Autodesk Fusion 360 part; units mm, degrees
sketch "Sketch2" plane through (0, 0, 0) normal (1, 0, 0) x (0, 1, 0)
  circle A0 centre (73.75, 0) radius 21.29
  line L0 (0, 0) -> (147.5, 0) construction
  circle A1 centre (73.75, 0) radius 18.75
  line L1 (78.83, -20.32) -> (78.83, -17.78)
  circle A2 centre (0, 0) radius 35.49
  line L2 (35.49, 0) -> (52.46, 0)
  circle A3 centre (46.6735, 34.4155) radius 22.5
  circle A4 centre (46.6735, -34.4155) radius 22.5
  circle A5 centre (0, 0) radius 32.95
  dimension "d11" = 37.5
  dimension "d14" = 2.54
  dimension "d24" = 65.9
  dimension "d25" = 2.54
  dimension "d26" = 73.75
  dimension "d27" = 45
extrude "Extrude2" add sketch "Sketch2" along normal blind 15.24 contours A0 | A0 A2 L2 A3 | A0 A2 L2 A4 | A2
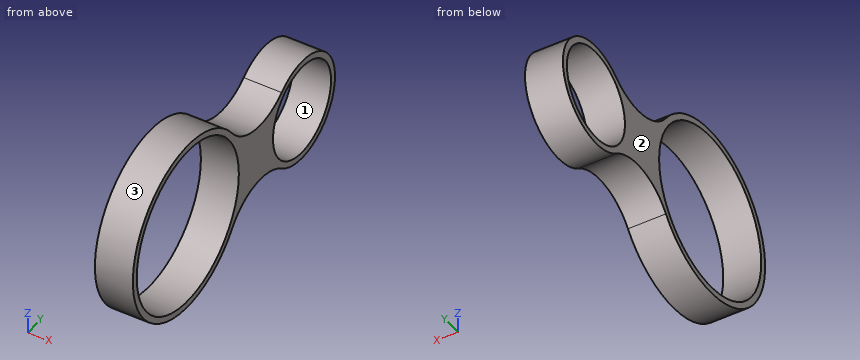
Can you work these out from the model? Positions are in its coordinate system, mm. Face numbers are marked on the shaded views. Give positions to 0.01 mm unless a question says otherwise; leave off trailing zeros. Loops run counter-clockwise (first coordinate to the right, second up) from the corner with the lowest first, then second, coordinate; pieces in that order, holes last. Notation, with made-up numbers: M -25.5,-21.75 L 26.5,-21.75 A24 ccw 26.5,9.25 Z; hole C -36.5,68 d9. An arc over 180 degrees is marked long. Use one line per item in the form item = value. Start each with the question number.
(1) I want a section at D-D, the plane x = 12.25. Write out the boundary of the cut face in (y, z), and give its area (3 significant figures).
(2) Thinking about a two-plate mould opening in Z: for the marked faces 1, 2 and 3, which applies, released by +Z, released by -Z, zero draft, split by the parting line, or undercut?
(3) I want a section at B-B, the plane y = 0. Write out the boundary of the cut face in (x, z), and give its area (3 significant figures).
(4) I'm going to push flat-ended pins straight in: P1, Ø6, axis at x = 10.5, z = 26, coming from the -Y side; P2, Ø3, axis at x = 4.5, y = 33, coming from the -Z side; P3, Ø6, axis at x = 9, z = -14, coming from the -Y side. Where does each tip first touch, or does it pass through?
(5) I want a section at C-C, the plane z = -27. Write out the boundary of the cut face in (x, y).
(6) I want a section at A-A, the plane z = 0. Write out the boundary of the cut face in (x, y), and give its area (3 significant figures).
(7) Please list where these lines run through material, in increasing order: line 1 (Z direction, x = 11.25, y = 73.75); line 2 (Z direction, x = 9.5, y = 0); line 3 (Y direction, x = 2, z = -11.5).
Worked out:
q1.outline = M 28.56,-21.06 A22.5 cw 60.59,-16.73 A21.29 ccw long 60.59,16.73 A22.5 cw 28.56,21.06 A35.49 ccw long Z; hole C 0,0 d65.9; hole C 73.75,0 d37.5
q1.area = 1,380 mm²
q2.face_1 = undercut
q2.face_2 = zero draft
q2.face_3 = split by the parting line
q3.outline = M 0,-35.49 L 15.24,-35.49 L 15.24,-32.95 L 0,-32.95 Z; M 0,32.95 L 15.24,32.95 L 15.24,35.49 L 0,35.49 Z
q3.area = 77.4 mm²
q4.P1 = -27.03
q4.P2 = -17.8
q4.P3 = -33.74
q5.outline = M 0,-23.03 L 15.24,-23.03 L 15.24,-18.89 L 0,-18.89 Z; M 0,18.89 L 15.24,18.89 L 15.24,23.03 L 0,23.03 Z
q6.outline = M 0,-35.49 L 15.24,-35.49 L 15.24,-32.95 L 0,-32.95 Z; M 0,32.95 L 15.24,32.95 L 15.24,55 L 0,55 Z; M 0,92.5 L 15.24,92.5 L 15.24,95.04 L 0,95.04 Z
q6.area = 413 mm²
q7.line_1 = -21.29 to -18.75, 18.75 to 21.29
q7.line_2 = -35.49 to -32.95, 32.95 to 35.49
q7.line_3 = -33.58 to -30.88, 30.88 to 58.94, 88.56 to 91.67
